The drawing under review shows one solid part. Ordinate dimensions are in mm from its lowest x, y, z. A direction names the side the tool comes from. Coordinates: 2 decimals unless noted, no trailing zeros. Write each loop counter-clockwise with the first axis right and the second up, starting at its lowest first coordinate (ties: lowest second). Pieces come first, ordered by that corner, then holes.
1) We need section C-C on z = 8.75. Write out the cut boundary in (x, y).
2) For the marked faces 1, 2 and 3, list the 3-axis set-ups (+Z, -Z, +X, -X, +Y, -Y) from which the entire face can be reached by the end or side of a thin tool; tool diameter is ignored.
3) To check wall thickness, follow line 1 along Z through (x, y) = (0.55, 0.5); line 2 along X through (y, z) = (2.15, 7.25); line 3 along X through (y, z) = (0.55, 8.5). State the ranges of each line that lie inside material, in increasing order.
4) We need section D-D on z = 2. Write out the cut boundary in (x, y), then the cut area to 3 significant figures.
5) We need section A-A on y = 1.55. Write out the cut boundary in (x, z), then the cut area to 4 significant figures.
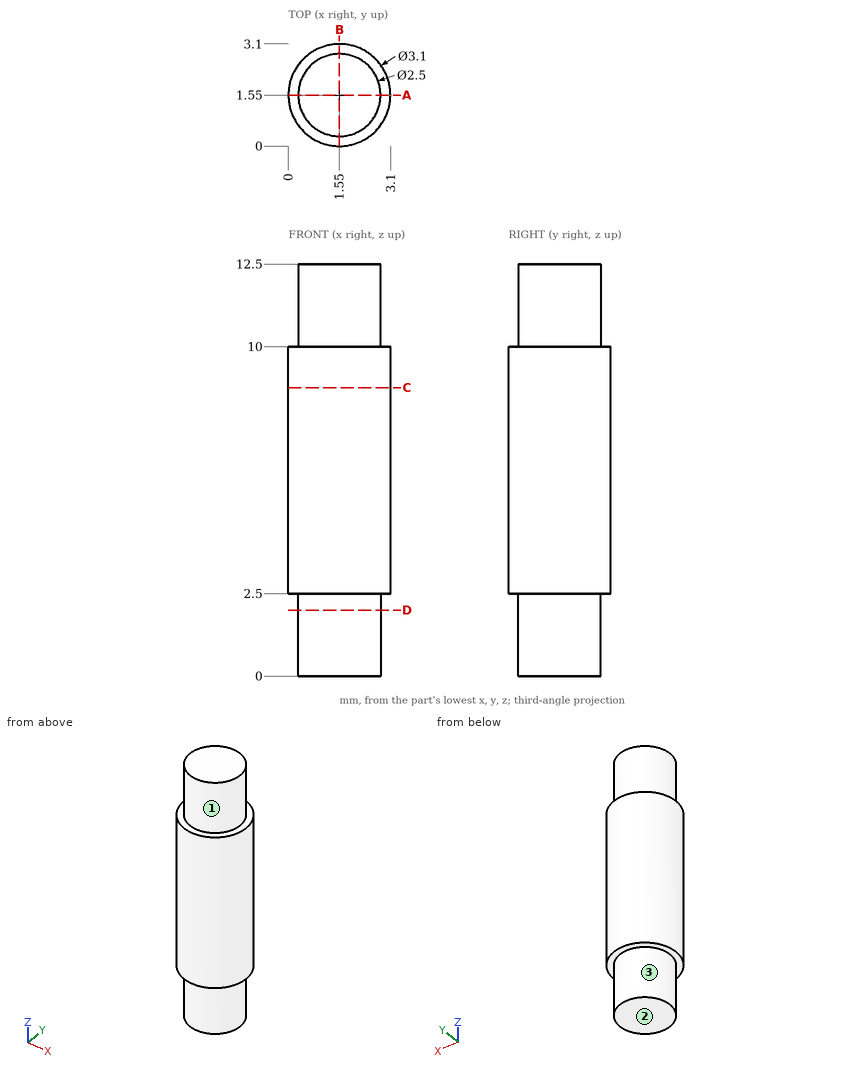
Result:
1. outline: circle Ø3.1 at (1.55, 1.55)
2. face 1: +Z
2. face 2: -Z, +X, -X, +Y, -Y
2. face 3: -Z
3. line 1: z = 2.5 to 10
3. line 2: x = 0.12 to 2.98
3. line 3: x = 0.37 to 2.73
4. outline: circle Ø2.5 at (1.55, 1.55)
4. area: 4.91 mm2
5. outline: (0, 2.5) - (0.3, 2.5) - (0.3, 0) - (2.8, 0) - (2.8, 2.5) - (3.1, 2.5) - (3.1, 10) - (2.8, 10) - (2.8, 12.5) - (0.3, 12.5) - (0.3, 10) - (0, 10) - close
5. area: 35.75 mm2
